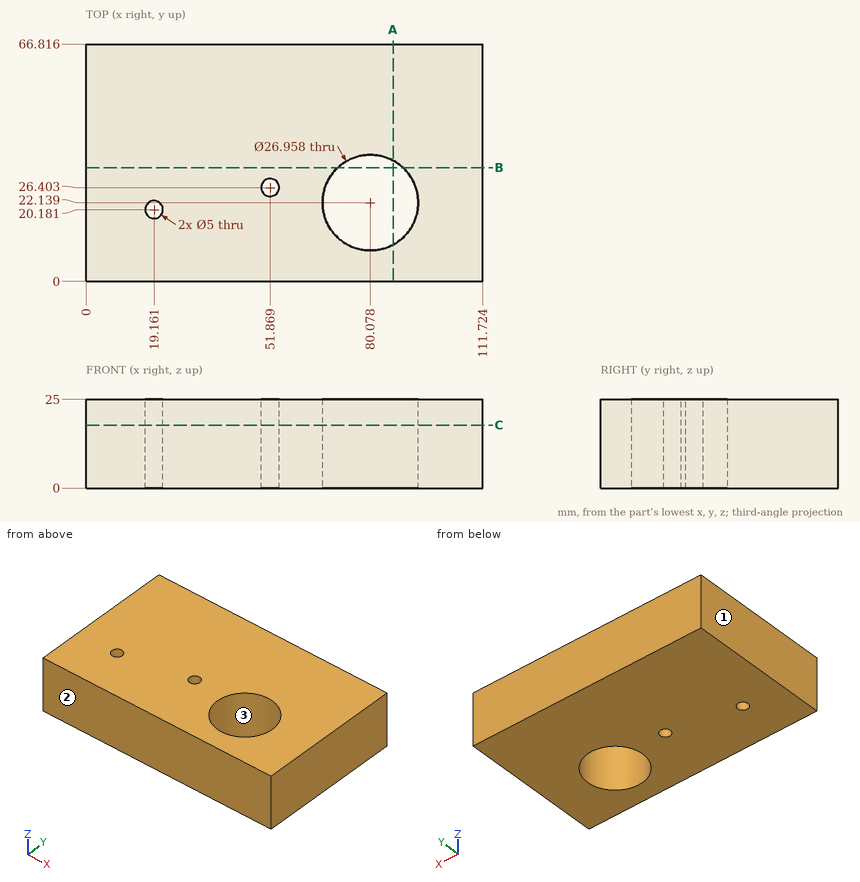
For this review, use the dimensioned drawing (mm, ordinates from the lowest corner) and the shaded views. Coordinates: 2 decimals unless noted, no trailing zeros. Loops run counter-clockwise (first coordinate to the right, second up) from the corner with the lowest first, then second, coordinate; pieces in that order, holes last. Notation, with made-up numbers: (-2.5, -11.5) - (17.5, -11.5) arc R16 ccw to (17.5, -1.5) - close; hole circle Ø3 at (75.25, 82). An arc over 180 degrees is marked (long way). Use CSV: the item, a comma, the result in double quotes. Start each with the question number.
1) Consider section B-B on y = 32. Write out the cut boundary in (x, z), then the cut area to 3 significant figures.
2) Consider section C-C on z = 17.75. Write out the cut boundary in (x, y).
3) Consider section A-A on x = 86.5. Write out the cut boundary in (y, z), then the cut area to 3 significant figures.
4) The part is to be moulded in two halves that separate along X. For the marked faces 1, 2 and 3, say which applies: +X half, -X half, draft (parallel to the pull), parting line (faces both ways), or undercut.
5) Wall thickness on L1, parallel to X at y = 21.5, z = 22 (1 decimal); L2, parallel to X at y = 27.5, z = 19.75 (1 decimal); L3, parallel to Y at x = 52, z = 21.5 (1 decimal): over which ranges is each line inside the solid? List them lowest first. Write a range as from..to.
Geometry says:
1,outline,"(0, 0) - (70.89, 0) - (70.89, 25) - (0, 25) - close; (89.27, 0) - (111.72, 0) - (111.72, 25) - (89.27, 25) - close"
1,area,"2,330 mm^2"
2,outline,"(0, 0) - (111.72, 0) - (111.72, 66.82) - (0, 66.82) - close; hole circle Ø5 at (19.16, 20.18); hole circle Ø5 at (51.87, 26.4); hole circle Ø26.96 at (80.08, 22.14)"
3,outline,"(0, 0) - (10.29, 0) - (10.29, 25) - (0, 25) - close; (33.99, 0) - (66.82, 0) - (66.82, 25) - (33.99, 25) - close"
3,area,"1,080 mm^2"
4,face 1,"-X half"
4,face 2,"draft"
4,face 3,"undercut"
5,L1,"0..17, 21.3..66.6, 93.5..111.7"
5,L2,"0..49.6, 54.1..67.7, 92.4..111.7"
5,L3,"0..23.9, 28.9..66.8"
